Autodesk Inventor part; units mm, degrees
ref_plane "YZ Plane" through (0, 0, 0) normal (1, 0, 0) x (0, 1, 0)
ref_plane "XZ Plane" through (0, 0, 0) normal (0, 1, 0) x (-1, 0, 0)
ref_plane "XY Plane" through (0, 0, 0) normal (0, 0, 1) x (1, 0, 0)
sketch "Sketch1" plane through (0, 0, 0) normal (0, 0, 1) x (1, 0, 0)
  circle A0 centre (0, 0) radius 100
  circle A1 centre (0, 0) radius 56
  circle A2 centre (0, 0) radius 67
  circle A3 centre (0, 0) radius 7.5
  dimension "d0" = 200
  dimension "d1" = 112
  dimension "d2" = 11
  dimension "d3" = 15
extrude "Extrusion1" add sketch "Sketch1" along normal mid plane 50 contours A0
extrude "Extrusion2" add sketch "Sketch1" along normal mid plane 85 contours A3
extrude "Extrusion3" add sketch "Sketch1" along normal mid plane 70 contours A1
extrude "Extrusion4" add sketch "Sketch1" along normal mid plane 40 contours A2
properties part number "motor at24v"
Check sheet for the modelled part. Datum: model origin and axes. Units: mm. A direction names the side the tool comes from. Give positions to 0.01 mm unless a question says otherwise; leave off trailing zeros. Loops run counter-clockwise (first coordinate to the right, second up) from the corner with the lowest first, then second, coordinate; pieces in that order, holes last. Notation, with made-up numbers: M 79.5,-7.75 L 106.5,-7.75 A24 cw 106.5,16.25 Z; hole C -13.75,9.5 d6. An arc over 180 degrees is marked long. Use a Markdown table: item, result. Add a question column.
Q1. Tool access check on faces 4 (the cylindrical face through (95.38, -30.04, -0.35)), 5 (the cylindrical face through (-7.493, 0.33, -38.698)), 6 (the flat face through (-15.2, -54.3, 20)). Record the directions out of +Z, -Z, +X, -X, +Y, -Y that give a thin tool (end or side, any length) a straight path to the whole face; none if there is none.
Q2. Mould release check, pull along X, two halves, no side actions. Record for faces 1 (the flat face through (21, -65, 25)), 2 (the cylindrical face through (-7.493, -0.33, 38.698)), 3 (the cylindrical face through (-14.524, -65.407, -22.465)): pulls with the +X half, pulls with the -X half, needs draft (parallel to the pull), parting line crosses it, or undercut.
Q3. Sectioned sample at D-D, the plane x = 52.5. Record the cut outline in (y, z), then the cut area to 3 significant figures.
Q4. Sectioned sample at A-A, the plane y = 0. Record the cut outline in (x, z), then the cut area to 3 significant figures.
Q5. Scan lines: line 1 along Y through (x, z) = (0, 21.75); line 2 along Z through (x, y) = (84.5, -37); line 3 along Z through (x, y) = (8.5, 63). Record each from-to range of solid material in increasing order. Write a range as [from, to].
Q6. Sectioned sample at C-C, the plane z = -2. Record the cut outline in (x, y), then the cut area to 3 significant figures.
Q7. Go/stop test with flat-tipped pins: pin 1 (10 mm diameter, centred on y = -38.5, z = 13.5, fed in from -X); pin 2 (3 mm diameter, centred on y = -60.5, z = 1.5, fed in from -X); pin 3 (5 mm diameter, centred on x = -68, z = -5, fed in from +Y); pin 4 (1.5 mm diameter, centred on y = 67.5, z = -26.5, fed in from +X). Record where each tip stops, or that it passes through.
Verdict:
| question | item | result |
|---|---|---|
| 1 | face 4 | +Z, -Z |
| 1 | face 5 | -Z |
| 1 | face 6 | +Z |
| 2 | face 1 | needs draft |
| 2 | face 2 | parting line crosses it |
| 2 | face 3 | undercut |
| 3 | outline | M -85.11,-25 L -41.63,-25 L -41.63,-20 L -19.49,-20 L -19.49,-35 L 19.49,-35 L 19.49,-20 L 41.63,-20 L 41.63,-25 L 85.11,-25 L 85.11,25 L 41.63,25 L 41.63,20 L 19.49,20 L 19.49,35 L -19.49,35 L -19.49,20 L -41.63,20 L -41.63,25 L -85.11,25 Z |
| 3 | area | 8,850 mm^2 |
| 4 | outline | M -100,-25 L -67,-25 L -67,-20 L -56,-20 L -56,-35 L -7.5,-35 L -7.5,-42.5 L 7.5,-42.5 L 7.5,-35 L 56,-35 L 56,-20 L 67,-20 L 67,-25 L 100,-25 L 100,25 L 67,25 L 67,20 L 56,20 L 56,35 L 7.5,35 L 7.5,42.5 L -7.5,42.5 L -7.5,35 L -56,35 L -56,20 L -67,20 L -67,25 L -100,25 Z |
| 4 | area | 12,200 mm^2 |
| 5 | line 1 | [-100, -67], [-56, 56], [67, 100] |
| 5 | line 2 | [-25, 25] |
| 5 | line 3 | [-20, 20] |
| 6 | outline | C 0,0 d200 |
| 6 | area | 31,400 mm^2 |
| 7 | pin 1 | x = -94.22 |
| 7 | pin 2 | x = -80.74 |
| 7 | pin 3 | y = 75.56 |
| 7 | pin 4 | through |
